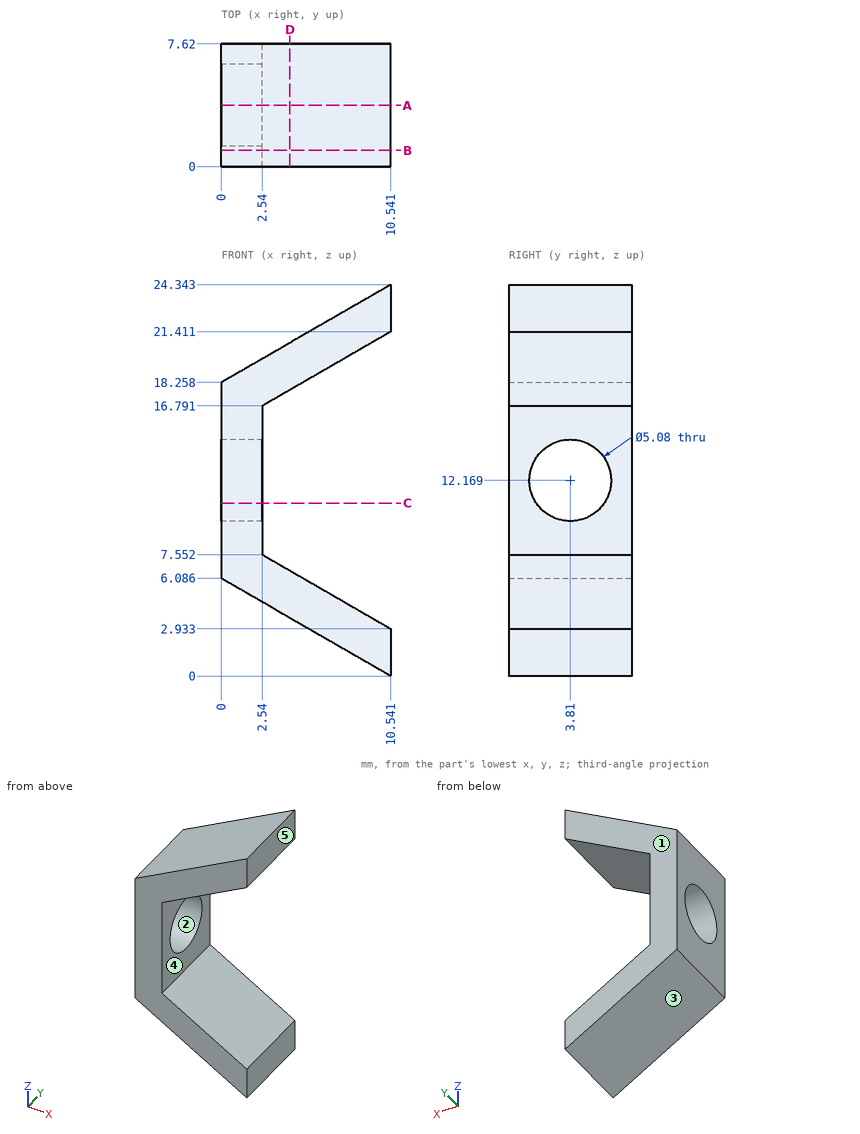
Drawing for the job (mm, zero at the part's lowest x, y, z). A direction names the side the tool comes from. Round coordinates to 2 decimals unless told otherwise and drop trailing zeros. Write each loop counter-clockwise with the first axis right and the second up, starting at its lowest first coordinate (ties: lowest second). Pieces come first, ordered by that corner, then holes. Notation, with made-up numbers: (89, 0) - (126, 0) arc R23 ccw to (126, 30) - close; hole circle Ø6 at (-26.5, 42). An arc over 180 degrees is marked (long way). Write item = value, one per line. Start each with the question number.
Q1. Mould opens along Z. For the marked faces 1, 2 and 3 say: pulls with the +Z half, pulls with the -Z half, needs draft (parallel to the pull), parting line crosses it, or undercut.
Q2. Probe L1, parallel to X at y = 6.5, z = 8; L2, parallel to Z at x = 1.75, y = 4.5 (1 decimal); L3, parallel to Z at x = 0.5, y = 5.75 (1 decimal). List the from-to ranges inside material, lowest first. Write a range as from..to.
Q3. Band-saw the part on A-A (y = 3.81). Give the cut face in (x, z) (1 decimal).
Q4. Band-saw the part on D-D (x = 4.25). Give the cut face in (y, z) (1 decimal).
Q5. Which spindle directions (+Z, -Z, +X, -X, +Y, -Y) get a long thin tool onto all of the face, cutting with end or side? Do the marked faces 4 and 5. Say none if no direction does.
Q6. Band-saw the part on C-C (z = 10.75). Give the cut face in (x, y).
Q7. Band-saw the part on B-B (y = 1). Give the cut face in (x, z) (1 decimal).
Q8. Drop a flat-ended pin along its axis: pin 1 (1 mm diameter, centred on y = 1, z = 14.5, fed in from +X). Give the stop position or say it passes through.
Answers below:
q1.face_1 = needs draft
q1.face_2 = undercut
q1.face_3 = pulls with the -Z half
q2.L1 = 0..2.54
q2.L2 = 5.1..9.7, 14.6..19.3
q2.L3 = 5.8..10.5, 13.8..18.5
q3.outline = (0, 6.1) - (10.5, 0) - (10.5, 2.9) - (2.5, 7.6) - (2.5, 9.6) - (0, 9.6) - close; (0, 14.7) - (2.5, 14.7) - (2.5, 16.8) - (10.5, 21.4) - (10.5, 24.3) - (0, 18.3) - close
q4.outline = (0, 3.6) - (7.6, 3.6) - (7.6, 6.6) - (0, 6.6) - close; (0, 17.8) - (7.6, 17.8) - (7.6, 20.7) - (0, 20.7) - close
q5.face_4 = +X, +Y, -Y
q5.face_5 = +Z, -Z, +X, +Y, -Y
q6.outline = (0, 0) - (2.54, 0) - (2.54, 1.7) - (0, 1.7) - close; (0, 5.92) - (2.54, 5.92) - (2.54, 7.62) - (0, 7.62) - close
q7.outline = (0, 6.1) - (10.5, 0) - (10.5, 2.9) - (2.5, 7.6) - (2.5, 16.8) - (10.5, 21.4) - (10.5, 24.3) - (0, 18.3) - close
q8.pin_1 = 2.54
